from build123d import *

# Parameters (mm, degrees)
F0_R     = 27
F0_R_2   = 21.97
F1_DEPTH = 29
F2_SIZE2 = 0.2886751346
F2_SIZE  = 0.5
F3_SIZE2 = 0.5773502692
F3_SIZE  = 1


with BuildPart() as f1:
    # F0 (on Top) → F1 (new body)
    with BuildSketch(Plane.XY):
        Circle(F0_R)
        Circle(F0_R_2, mode=Mode.SUBTRACT)
    extrude(amount=F1_DEPTH)

    # F2
    f2_edges = [f1.edges().sort_by_distance(p)[0] for p in [
        (-27, 0, 29),
        (-27, 0, 0),
    ]]
    f2_side = f1.faces().sort_by_distance((-27, 0, 14.5))[0]
    chamfer(f2_edges, length=F2_SIZE, length2=F2_SIZE2, reference=f2_side)

    # F3
    f3_edges = [f1.edges().sort_by_distance(p)[0] for p in [
        (-21.97, 0, 0),
    ]]
    f3_side = f1.faces().sort_by_distance((-21.97, 0, 14.5))[0]
    chamfer(f3_edges, length=F3_SIZE, length2=F3_SIZE2, reference=f3_side)

    # F4 (on Front) → F5 (revolve, cut)
    with BuildSketch(Plane.XZ):
        Polygon((-22.2379491924, 28), (-21.97, 27), (-21.97, 29), (-23.2379491924, 29), align=None)
    revolve(axis=Axis((0, 0, 15.0005389005), (0, 0, -1)), mode=Mode.SUBTRACT)


solid = f1.part
For this review, take the finished solid that the model builds, in its own axes (mm). Round coordinates to 2 decimals unless told otherwise and drop trailing zeros. Order: outer loops, then holes, each group sorted by start corner. A loop starts at its lowest first (then second) coordinate and runs counter-clockwise, first axis right, second up. Notation, with made-up numbers: (57.5, -15) -> (63.5, -15) arc R19 cw to (63.5, 7) -> close; hole circle Ø4 at (-1.75, 2.5). An arc over 180 degrees is marked (long way). Write item = value, one per line. Start each with the question number.
1) To check wall thickness, follow line 1 (Y direction, x = 0, z = 11.25); line 2 (X direction, y = 12.5, z = 18.75); line 3 (X direction, y = -8.5, z = 6). State the ranges of each line that lie inside material, in increasing order. Write a range as from..to.
2) Take a section at A-A on x = 0. State the section outline as (y, z) points.
3) The part is to be moulded in two halves that separate along Y. For faces 1 (the face through (-18, -14, 0)), 2 (the face through (-4.76, -21.45, 13.82)), 3 (the face through (-5.85, -26.36, 14.3)), say which applies: +Y half, -Y half, draft (parallel to the pull), parting line (faces both ways), or undercut.
4) Insertion check: pin 1 (5 mm diameter, centred on y = -6, z = 10, fed in from +X); pin 2 (2 mm diameter, centred on x = 17, y = -12, fed in from -Z); pin 3 (3 mm diameter, centred on x = -17.5, z = 3.5, fed in from +Y); pin 4 (1 mm diameter, centred on x = -9, z = 22, fed in from +Y). Each pin has a flat end and moves straight along its axis. Give the tip position at first contact, or say it passes through.
5) Take a section at C-C on z = 2. State the section outline as (x, y) points, plus the area to 3 significant figures.
Verdict:
q1.line_1 = -27..-21.97, 21.97..27
q1.line_2 = -23.93..-18.07, 18.07..23.93
q1.line_3 = -25.63..-20.26, 20.26..25.63
q2.outline = (-27, 0.5) -> (-26.71, 0) -> (-22.55, 0) -> (-21.97, 1) -> (-21.97, 27) -> (-22.24, 28) -> (-23.24, 29) -> (-26.71, 29) -> (-27, 28.5) -> close; (21.97, 1) -> (22.55, 0) -> (26.71, 0) -> (27, 0.5) -> (27, 28.5) -> (26.71, 29) -> (23.24, 29) -> (22.24, 28) -> (21.97, 27) -> close
q3.face_1 = draft
q3.face_2 = undercut
q3.face_3 = parting line
q4.pin_1 = 26.77
q4.pin_2 = through
q4.pin_3 = 21.75
q4.pin_4 = 25.63
q5.outline = circle Ø54 at (0, 0); hole circle Ø43.94 at (0, 0)
q5.area = 774 mm2
